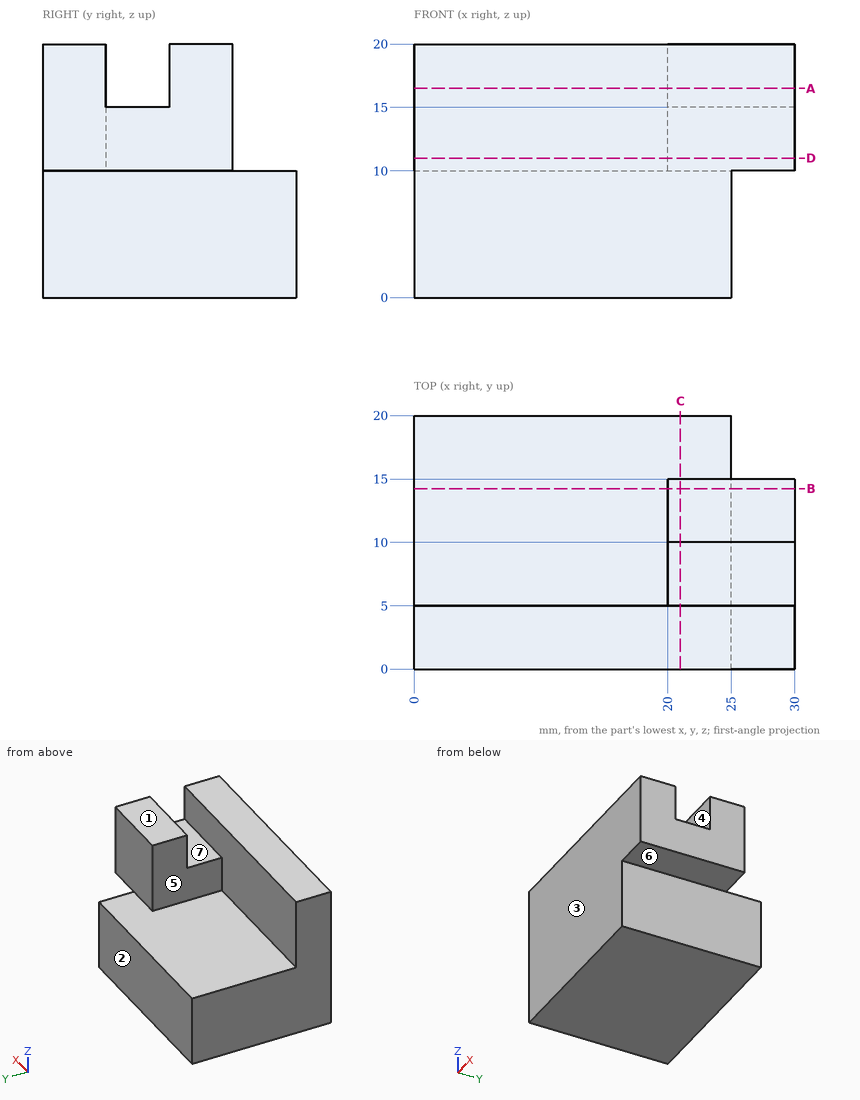
Source: three-view drawing plus pictorial views. Frame: mm from the lowest corner of the part. A direction names the side the tool comes from. Give positions to 0.01 mm unless a question says otherwise; leave off trailing zeros. Order: outer loops, then holes, each group sorted by start corner. A loop starts at its lowest first (then second) coordinate and runs counter-clockwise, first axis right, second up. Notation, with made-up numbers: M 2,70 L 30,70 A29 cw 30,94 Z; hole C 47.25,-28.75 d3. An arc over 180 degrees is marked long. Return JSON: item names as keys, results as strings.
Item 1: Cut plane D-D (z = 11). Return loops of the section in (x, y).
Solutions:
{"outline": "M 0,0 L 30,0 L 30,15 L 20,15 L 20,5 L 0,5 Z"}
Item 2: Cut plane C-C (x = 21). Return loops of the section in (y, z).
Solutions:
{"outline": "M 0,0 L 20,0 L 20,10 L 15,10 L 15,20 L 10,20 L 10,15 L 5,15 L 5,20 L 0,20 Z"}
Item 3: First-contact query: P1, Ø7.5, axis at x = 7.5, y = 16, coming from the +Z side; P2, Ø8, axis at y = 11.5, z = 18, coming from the -X side; P3, Ø3, axis at x = 19.5, z = 17.5, coming from the +Y side. Flat tips, straight axial feed; report the tip coordinate or a pass-through.
Solutions:
{"P1": "z = 10", "P2": "x = 20", "P3": "y = 15"}
Item 4: Cut plane B-B (y = 14.25). Return loops of the section in (x, z), then the cut area to 3 significant figures.
Solutions:
{"outline": "M 0,0 L 25,0 L 25,10 L 30,10 L 30,20 L 20,20 L 20,10 L 0,10 Z", "area": "350 mm^2"}
Item 5: Ray query, probe 1 along Z at (x, y) = (27, 3.5); probe 2 along X at (y, z) = (3, 5.25); probe 3 along Y at (x, z) = (24.25, 12). Return the intervals inside material, ascending.
Solutions:
{"probe 1": "10 to 20", "probe 2": "0 to 25", "probe 3": "0 to 15"}
Item 6: Pull-direction query (Y, two-part tool) for the marked faces 1, 2, 3 and 4; classes: +Y half, -Y half, draft (parallel to the pull), parting line (faces both ways), or undercut.
Solutions:
{"face 1": "draft", "face 2": "+Y half", "face 3": "-Y half", "face 4": "undercut"}
Item 7: Access query for the marked faces 5, 6 and 7. Directions: +Z, -Z, +X, -X, +Y, -Y. A direction counts if a zero-diameter tool reaches every point of the face in a straight line with its end or side. Return the directions, or none.
Solutions:
{"face 5": "+Z, -X, +Y", "face 6": "-Z, +X, +Y, -Y", "face 7": "+Z, +X, -X"}
Item 8: Cut plane A-A (z = 16.5). Return loops of the section in (x, y).
Solutions:
{"outline": "M 0,0 L 30,0 L 30,5 L 0,5 Z; M 20,10 L 30,10 L 30,15 L 20,15 Z"}
